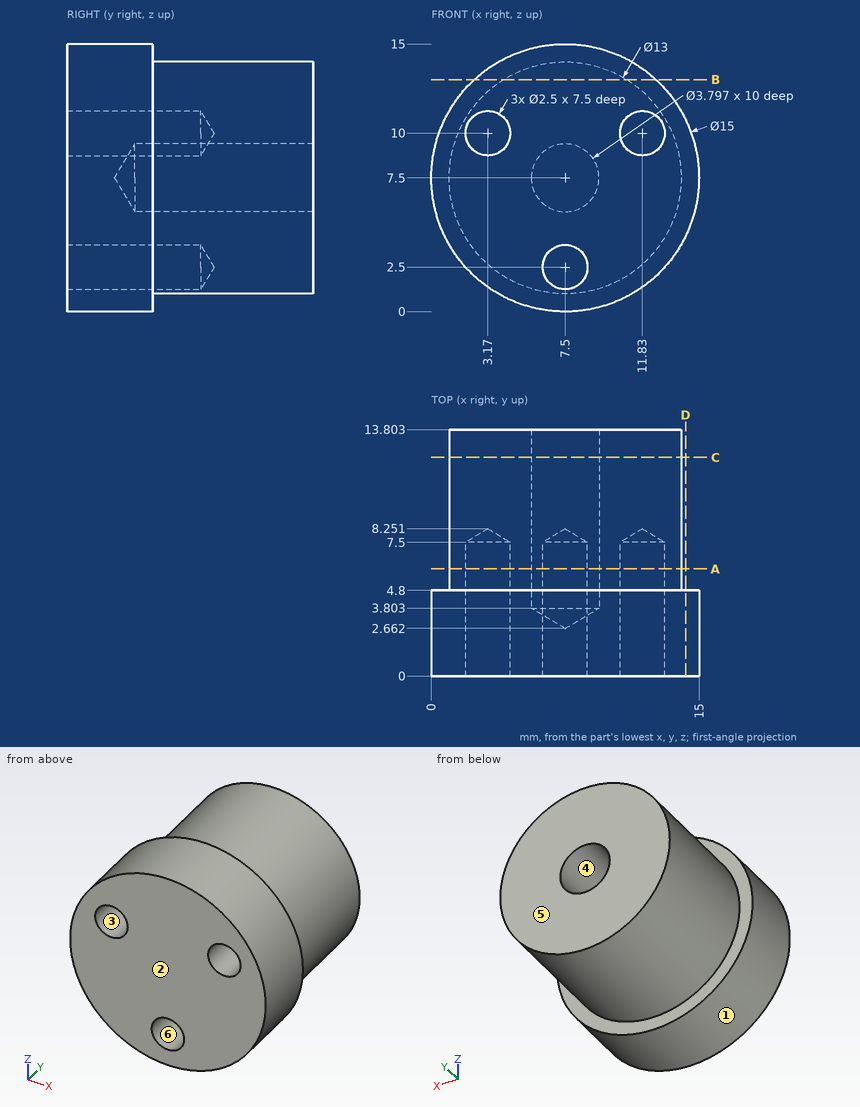
Verification items for this drawing (mm, ordinates from the low corner). A direction names the side the tool comes from. Coordinates: 2 decimals unless noted, no trailing zeros. Order: outer loops, then holes, each group sorted by start corner. A loop starts at its lowest first (then second) coordinate and runs counter-clockwise, first axis right, second up. Notation, with made-up numbers: (24.25, 60) -> (39.25, 60) arc R19 ccw to (39.25, 95) -> close; hole circle Ø1 at (86, 78). An arc over 180 degrees is marked (long way). Answer as CSV lines item,"result". Start each with the question number.
1) Cross-section at D-D, the plane x = 14.25. Record the boundary of the cut face in (y, z).
2) Set-up check for the marked faces 4, 5 and 6: record each of +Z, -Z, +X, -X, +Y, -Y from which the full face is reachable in a straight line by a thin tool's end or side.
3) Cross-section at B-B, the plane z = 13. Record the boundary of the cut face in (x, y) (1 decimal), then the cut area to 3 significant figures.
4) Gauge pin test, flat ends, axial feed: pin 1 Ø3 at (x, z) = (3.17, 10) entering from -Y; pin 2 Ø2 at (y, z) = (6, 5) entering from +X (1 decimal); pin 3 Ø5 at (x, y) = (4.5, 2) entering from -Z; pin 4 Ø3 at (y, z) = (6.5, 4.5) entering from -X (1 decimal). Record the tip position at first contact, or that the pin passes through.
5) Release check for a two-part mould opening along X. For the marked faces 1, 2 and 3 record: released by +X, released by -X, zero draft, split by the parting line, or undercut.
6) Material ranges on L1, parallel to Z at x = 7.5, y = 4; L2, parallel to Z at x = 7.5, y = 7; L3, parallel to Z at x = 7.5, y = 8.5, recorded low to high. Write a range as [from, to].
7) Cross-section at A-A, the plane y = 6. Record the boundary of the cut face in (x, z).
8) Cross-section at C-C, the plane y = 12.25. Record the boundary of the cut face in (x, z).
Conclusion:
1,outline,"(0, 4.23) -> (4.8, 4.23) -> (4.8, 10.77) -> (0, 10.77) -> close"
2,face 4,"+Y"
2,face 5,"+Z, -Z, +X, -X, +Y"
2,face 6,"-Y"
3,outline,"(2.4, 0) -> (12.6, 0) -> (12.6, 4.8) -> (11, 4.8) -> (11, 13.8) -> (4, 13.8) -> (4, 4.8) -> (2.4, 4.8) -> close"
3,area,"111 mm²"
4,pin 1,"stops at y = 0"
4,pin 2,"stops at x = 13.8"
4,pin 3,"stops at z = 0.02"
4,pin 4,"stops at x = 1.2"
5,face 1,"split by the parting line"
5,face 2,"zero draft"
5,face 3,"undercut"
6,L1,"z = [0, 1.25], [3.75, 5.6], [9.4, 15]"
6,L2,"z = [1, 1.25], [3.75, 5.6], [9.4, 14]"
6,L3,"z = [1, 5.6], [9.4, 14]"
7,outline,"circle Ø13 at (7.5, 7.5); hole circle Ø2.5 at (3.17, 10); hole circle Ø3.8 at (7.5, 7.5); hole circle Ø2.5 at (7.5, 2.5); hole circle Ø2.5 at (11.83, 10)"
8,outline,"circle Ø13 at (7.5, 7.5); hole circle Ø3.8 at (7.5, 7.5)"
